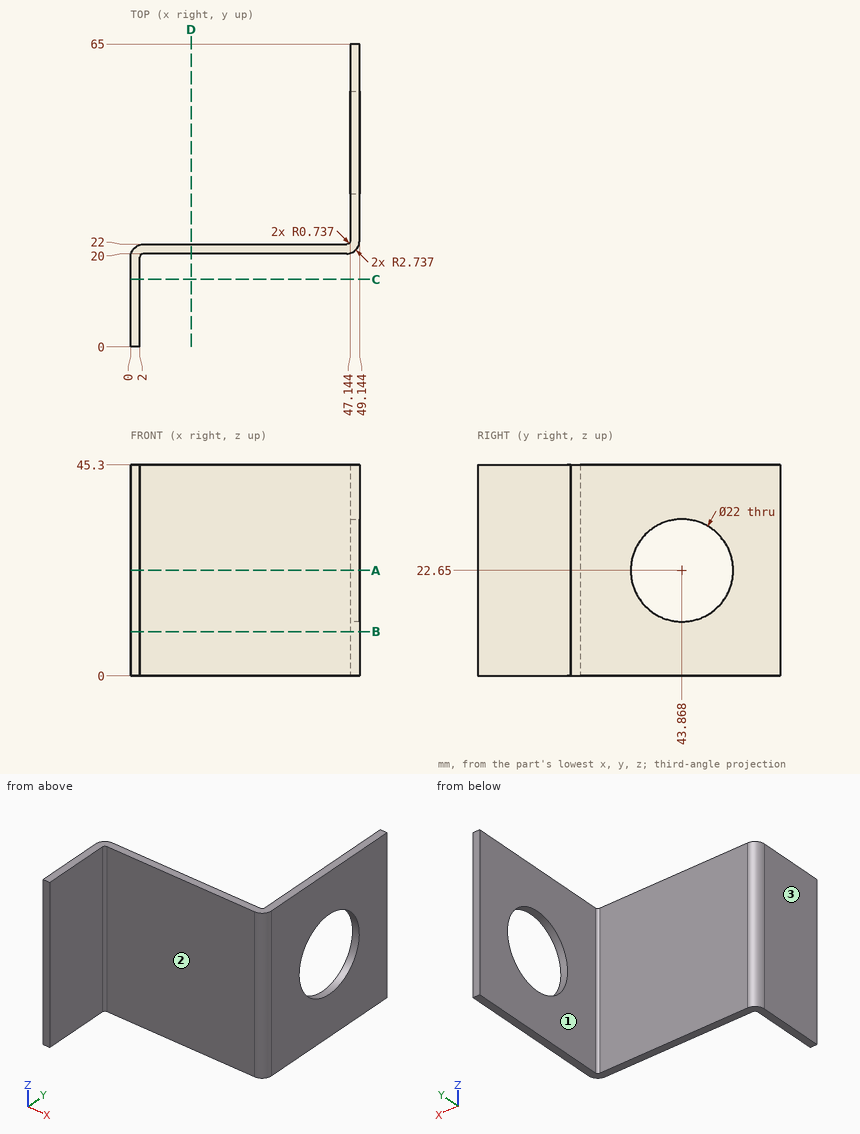
Geometry: see drawing. Coordinates: mm, zero at the bounding-box minimum. A direction names the side the tool comes from. Coordinates: 2 decimals unless noted, no trailing zeros. Order: outer loops, then holes, each group sorted by start corner. A loop starts at its lowest first (then second) coordinate and runs counter-clockwise, first axis right, second up. Notation, with made-up numbers: M 53,-19 L 90,-19 A24 ccw 90,8 Z; hole C -19.5,63 d9. An arc over 180 degrees is marked long. Answer in a Markdown table with one row per item. Add a question column.
Q1. Section query A-A on z = 22.65. Return the cut outline in (x, y).
Q2. Contact query for flat-ended pins moving along their axis: P1, Ø12, axis at y = 37, z = 9, coming from the -X side; P2, Ø15.5, axis at y = 13, z = 15, coming from the +X side; P3, Ø10, axis at x = 9, z = 23.5, coming from the -Y side. Output: stop coordinate, or through.
Q3. Reachability of the marked faces 1, 2 and 3 from +Z, -Z, +X, -X, +Y, -Y: full face, straight path, thin tool, end or side. Return the list, or none.
Q4. Section query C-C on y = 14.5. Return the cut outline in (x, z).
Q5. Section query B-B on z = 9.5. Return the cut outline in (x, y), and give its area (3 significant figures).
Q6. Section query D-D on x = 13. Return the cut outline in (y, z).
Q7. Line query: L1, parallel to X at y = 6, z = 2.5; L2, parallel to Y at x = 30.5, z = 17; L3, parallel to X at y = 24, z = 19. Output: solid intervals per line, ascending.
Completed:
| question | item | result |
|---|---|---|
| 1 | outline | M 0,0 L 2,0 L 2,19.26 A0.74 cw 2.74,20 L 46.41,20 A2.74 ccw 49.14,22.74 L 49.14,32.87 L 47.14,32.87 L 47.14,22.74 A0.74 cw 46.41,22 L 2.74,22 A2.74 ccw 0,19.26 Z; M 47.14,54.87 L 49.14,54.87 L 49.14,65 L 47.14,65 Z |
| 2 | P1 | stops at x = 47.14 |
| 2 | P2 | stops at x = 48.29 |
| 2 | P3 | stops at y = 20 |
| 3 | face 1 | +Z, -Z, -X, +Y |
| 3 | face 2 | +Z, -Z, +X, -Y |
| 3 | face 3 | +Z, -Z, -X, +Y, -Y |
| 4 | outline | M 0,0 L 2,0 L 2,45.3 L 0,45.3 Z |
| 5 | outline | M 0,0 L 2,0 L 2,19.26 A0.74 cw 2.74,20 L 46.41,20 A2.74 ccw 49.14,22.74 L 49.14,65 L 47.14,65 L 47.14,22.74 A0.74 cw 46.41,22 L 2.74,22 A2.74 ccw 0,19.26 Z |
| 5 | area | 221 mm2 |
| 6 | outline | M 20,0 L 22,0 L 22,45.3 L 20,45.3 Z |
| 7 | L1 | x = 0 to 2 |
| 7 | L2 | y = 20 to 22 |
| 7 | L3 | x = 47.14 to 49.14 |
